Verification items for the finished model (mm, model axes). Face numbers are marked on the shaded views. A direction names the side the tool comes from. Round coordinates to 2 decimals unless told otherwise and drop trailing zeros. Loops run counter-clockwise (first coordinate to the right, second up) from the corner with the lowest first, then second, coordinate; pieces in that order, holes last.
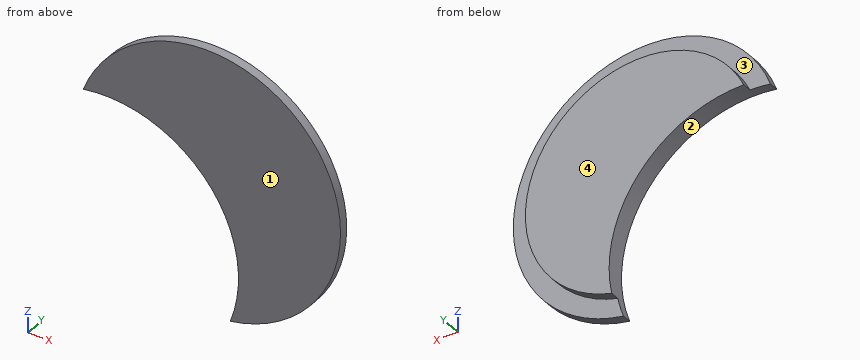
from build123d import *

# Parameters (mm, degrees)
F0_R     = 37.5
F1_DEPTH = 3
F2_R     = 43.5
F3_DEPTH = 3
F5_DEPTH = 25


with BuildPart() as f1:
    # F0 (on Front) → F1 (new body)
    with BuildSketch(Plane.XZ):
        Circle(F0_R)
    extrude(amount=F1_DEPTH)

    # F2 (on face) → F3 (join)
    with BuildSketch(Plane.XZ.offset(3)):
        Circle(F2_R)
    extrude(amount=F3_DEPTH)

    # F4 (on face) → F5 (cut)
    with BuildSketch(Plane(origin=(0, 0, 0), x_dir=(-1, 0, 0), z_dir=(0, 1, 0))):
        with BuildLine():
            ThreePointArc((40.8147967737, 15.0466728654), (0, 0), (-7.376597443, -42.8699872891))
            ThreePointArc((-7.376597443, -42.8699872891), (33.4381993307, -27.8233144237), (40.8147967737, 15.0466728654))
        make_face()
    extrude(amount=-F5_DEPTH, mode=Mode.SUBTRACT)


solid = f1.part
1. Section check D-D (x = 0). Enter the section's corners in (y, z).
2. Section check B-B (z = 31.5). Enter the section's corners in (x, y), then the cut area to 3 significant figures.
3. Tool access check on the marked faces 3 and 4. Record the directions out of +Z, -Z, +X, -X, +Y, -Y that give a thin tool (end or side, any length) a straight path to the whole face; none if there is none.
4. Section check C-C (z = 0). Enter the section's corners in (x, y), then the cut area to 3 significant figures.
5. Scan lines: L1, parallel to Y at x = 21.5, z = -36; L2, parallel to X at y = -2.2, z = 0; L3, parallel to Z at x = 35, y = -4.5. Record each from-to range of solid material in increasing order.
6. Release check for a two-part mould opening along Z. For the marked faces 1 and 2 record: released by +Z, released by -Z, zero draft, split by the parting line, or undercut.
7. Section check A-A (x = 12). Enter the section's corners in (y, z).
8. Gauge pin test, flat ends, axial feed: P1, Ø1, axis at x = 19, y = -4, coming from the +Z side; P2, Ø1.5, axis at y = -5, z = 11, coming from the +X side. Record the tip position at first contact, or that the pin passes through.
Taken from the geometry:
1. outline: (-6, 0) - (0, 0) - (0, 37.5) - (-3, 37.5) - (-3, 43.5) - (-6, 43.5) - close
2. outline: (-30, -6) - (30, -6) - (30, -3) - (20.35, -3) - (20.35, 0) - (-20.35, 0) - (-20.35, -3) - (-30, -3) - close
2. area: 302 mm2
3. face 3: +Y
3. face 4: +Z, -Z, +X, -X, +Y
4. outline: (0, -6) - (43.5, -6) - (43.5, -3) - (37.5, -3) - (37.5, 0) - (0, 0) - close
4. area: 243 mm2
5. L1: y = -6 to -3
5. L2: x = 0 to 37.5
5. L3: z = -25.83 to 25.83
6. face 1: zero draft
6. face 2: undercut
7. outline: (-6, -41.81) - (-3, -41.81) - (-3, -35.53) - (0, -35.53) - (0, 35.53) - (-3, 35.53) - (-3, 41.81) - (-6, 41.81) - close
8. P1: stops at z = 39.37
8. P2: stops at x = 42.28
